Check sheet for the modelled part. Datum: model origin and axes. Units: mm. Face numbers are marked on the shaded views. A direction names the side the tool comes from. Coordinates: 2 decimals unless noted, no trailing zeros. Order: outer loops, then holes, each group sorted by start corner. A loop starts at its lowest first (then second) coordinate and runs counter-clockwise, first axis right, second up.
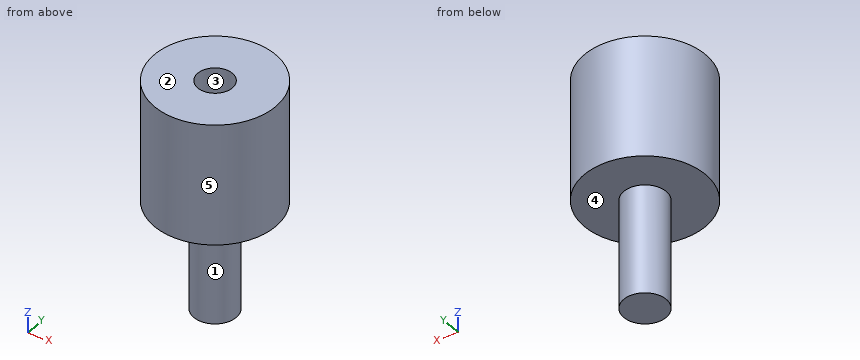
Autodesk Inventor part; units mm, degrees
ref_plane "YZ Plane" through (0, 0, 0) normal (1, 0, 0) x (0, 1, 0)
ref_plane "XZ Plane" through (0, 0, 0) normal (0, 1, 0) x (-1, 0, 0)
ref_plane "XY Plane" through (0, 0, 0) normal (0, 0, 1) x (1, 0, 0)
sketch "Sketch7" plane through (0, 0, 0) normal (0, 0, 1) x (1, 0, 0)
  circle A0 centre (0, 0) radius 1.75
  dimension "d19" = 3.5
extrude "Extrusion6" add sketch "Sketch7" along normal blind 9
sketch "Sketch8" plane through (0, 0, 9) normal (0, 0, 1) x (1, 0, 0)
  circle A0 centre (0, 0) radius 5
  dimension "d22" = 10
extrude "Extrusion7" add sketch "Sketch8" along normal blind 10
sketch "Sketch9" plane through (0, 0, 19) normal (0, 0, 1) x (1, 0, 0)
  point P0 (0, 0)
  point P1 (0, 0)
hole "Hole1" at (0, 0, 19) direction (0, 0, -1) diameter 2.85 depth 8
properties part number "Elbow_Parallel_Rod_V1"
(1) Thickness scan on probe 1 along Y at (x, z) = (0, 16.5) (3 decimals); probe 2 along Z at (x, y) = (-0.5, 0); probe 3 along Z at (x, y) = (4.25, -1.25). Record the ranges inside material, lowest first.
Filled in:
probe 1: y = -5 to -1.425, 1.425 to 5
probe 2: z = 0 to 11
probe 3: z = 9 to 19
(2) Cross-section at A-A (y = 0). Enter the section's corners in (x, z) (3 decimals).
Filled in:
outline: (-5, 9) - (-1.75, 9) - (-1.75, 0) - (1.75, 0) - (1.75, 9) - (5, 9) - (5, 19) - (1.425, 19) - (1.425, 11) - (-1.425, 11) - (-1.425, 19) - (-5, 19) - close
(3) Tool access check on the marked faces 4 and 5. Record the directions out of +Z, -Z, +X, -X, +Y, -Y that give a thin tool (end or side, any length) a straight path to the whole face; none if there is none.
Filled in:
face 4: -Z
face 5: +Z, -Z
(4) Cross-section at C-C (z = 11.5). Enter the section's corners in (x, y) (3 decimals), and give its area (3 significant figures).
Filled in:
outline: circle Ø10 at (0, 0); hole circle Ø2.85 at (0, 0)
area: 72.2 mm2
(5) Go/stop test with flat-tipped pins: P1, Ø2, axis at y = -0.5, z = 16, coming from the -X side; P2, Ø1.4, axis at x = -0.5, y = 0, coming from the +Z side; P3, Ø3, axis at x = 2.5, z = 2, coming from the -Y side; P4, Ø3, axis at y = -3, z = 16, coming from the +X side. Record where each tip stops, or that it passes through.
Filled in:
P1: stops at x = -5
P2: stops at z = 11
P3: stops at y = -1.44
P4: stops at x = 4.77
(6) Cross-section at D-D (y = -4). Enter the section's corners in (x, z).
Filled in:
outline: (-3, 9) - (3, 9) - (3, 19) - (-3, 19) - close
(7) Release check for a two-part mould opening along X. For the marked faces 1, 2 and 3 record: +X half, -X half, draft (parallel to the pull), parting line (faces both ways), or undercut.
Filled in:
face 1: parting line
face 2: draft
face 3: undercut
